from build123d import *

# Parameters (mm, degrees)
BOSS_EXTRUDE1_DEPTH = 5
SKETCH1_3_R         = 2.1
CUT_EXTRUDE1_DEPTH  = 57.124860802
SKETCH1_4_R         = 2.1
CUT_EXTRUDE2_DEPTH  = 57.124860802
SKETCH1_5_R         = 2.1
CUT_EXTRUDE3_DEPTH  = 57.124860802
SKETCH1_6_R         = 2.1
CUT_EXTRUDE4_DEPTH  = 57.124860802
BOSS_EXTRUDE2_DEPTH = 6
FILLET1_R           = 2
FILLET2_R           = 2
FILLET3_R           = 2
FILLET4_R           = 2
FILLET5_R           = 1


with BuildPart() as part:
    # Sketch1 → Boss-Extrude1 (new body)
    with BuildSketch(Plane(origin=(0, 0, 0), x_dir=(1, 0, 0), z_dir=(0, 1, 0))):
        with BuildLine():
            Line((-20, 0), (20, 0))
            ThreePointArc((20, 0), (23.535533906, -1.464466094), (25, -5))
            Line((25, -5), (25, -45))
            ThreePointArc((25, -45), (23.535533906, -48.535533906), (20, -50))
            Line((20, -50), (-20, -50))
            ThreePointArc((-20, -50), (-23.535533906, -48.535533906), (-25, -45))
            Line((-25, -45), (-25, -5))
            ThreePointArc((-25, -5), (-23.535533906, -1.464466094), (-20, 0))
        make_face()
    extrude(amount=BOSS_EXTRUDE1_DEPTH)

    # Sketch1_3 → Cut-Extrude1 (cut, through all)
    with BuildSketch(Plane(origin=(0, 0, 0), x_dir=(1, 0, 0), z_dir=(0, 1, 0))):
        with Locations(Location((20, -45, 0), (0, 0, 270))):
            Circle(SKETCH1_3_R)
    extrude(amount=CUT_EXTRUDE1_DEPTH, mode=Mode.SUBTRACT)

    # Sketch1_4 → Cut-Extrude2 (cut, through all)
    with BuildSketch(Plane(origin=(0, 0, 0), x_dir=(1, 0, 0), z_dir=(0, 1, 0))):
        with Locations(Location((20, -5, 0), (0, 0, 270))):
            Circle(SKETCH1_4_R)
    extrude(amount=CUT_EXTRUDE2_DEPTH, mode=Mode.SUBTRACT)

    # Sketch1_5 → Cut-Extrude3 (cut, through all)
    with BuildSketch(Plane(origin=(0, 0, 0), x_dir=(1, 0, 0), z_dir=(0, 1, 0))):
        with Locations(Location((-20, -5, 0), (0, 0, 90))):
            Circle(SKETCH1_5_R)
    extrude(amount=CUT_EXTRUDE3_DEPTH, mode=Mode.SUBTRACT)

    # Sketch1_6 → Cut-Extrude4 (cut, through all)
    with BuildSketch(Plane(origin=(0, 0, 0), x_dir=(1, 0, 0), z_dir=(0, 1, 0))):
        with Locations(Location((-20, -45, 0), (0, 0, 90))):
            Circle(SKETCH1_6_R)
    extrude(amount=CUT_EXTRUDE4_DEPTH, mode=Mode.SUBTRACT)

    # Sketch1_8 → Boss-Extrude2 (add)
    with BuildSketch(Plane(origin=(0, 0, 0), x_dir=(1, 0, 0), z_dir=(0, 1, 0))):
        with BuildLine():
            Line((17.051994501, -27.070918511), (17.051994501, -16.496039026))
            Line((17.051994501, -16.496039026), (20.029081489, -16.496039026))
            Line((20.029081489, -16.496039026), (20.029081489, -27.070918511))
            ThreePointArc((20.029081489, -27.070918511), (0, -47.1), (-20.029081489, -27.070918511))
            Line((-20.029081489, -27.070918511), (-20.029081489, -16.496039026))
            Line((-20.029081489, -16.496039026), (-17.051994501, -16.496039026))
            Line((-17.051994501, -16.496039026), (-17.051994501, -27.070918511))
            ThreePointArc((-17.051994501, -27.070918511), (0, -44.122913013), (17.051994501, -27.070918511))
        make_face()
    extrude(amount=-BOSS_EXTRUDE2_DEPTH)

    # Fillet1
    fillet1_edges = [part.edges().sort_by_distance(p)[0] for p in [
        (20.029081489, 0, 21.783478769),
        (-20.029081489, 0, 21.783478769),
        (0, 0, 47.1),
    ]]
    fillet(fillet1_edges, radius=FILLET1_R)

    # Fillet2
    fillet2_edges = [part.edges().sort_by_distance(p)[0] for p in [
        (17.051994501, -3, 16.496039026),
    ]]
    fillet(fillet2_edges, radius=FILLET2_R)

    # Fillet3
    fillet3_edges = [part.edges().sort_by_distance(p)[0] for p in [
        (-17.051994501, -3, 16.496039026),
    ]]
    fillet(fillet3_edges, radius=FILLET3_R)

    # Fillet4
    fillet4_edges = [part.edges().sort_by_distance(p)[0] for p in [
        (-20.029081489, -6, 21.783478769),
        (0, -6, 47.1),
        (20.029081489, -6, 21.783478769),
    ]]
    fillet(fillet4_edges, radius=FILLET4_R)

    # Fillet5
    fillet5_edges = [part.edges().sort_by_distance(p)[0] for p in [
        (0, 0, 0),
        (-23.535533906, 0, 1.464466094),
        (-25, 0, 25),
        (-23.535533906, 0, 48.535533906),
        (0, 0, 50),
        (23.535533906, 0, 48.535533906),
        (25, 0, 25),
        (23.535533906, 0, 1.464466094),
    ]]
    fillet(fillet5_edges, radius=FILLET5_R)


solid = part.part
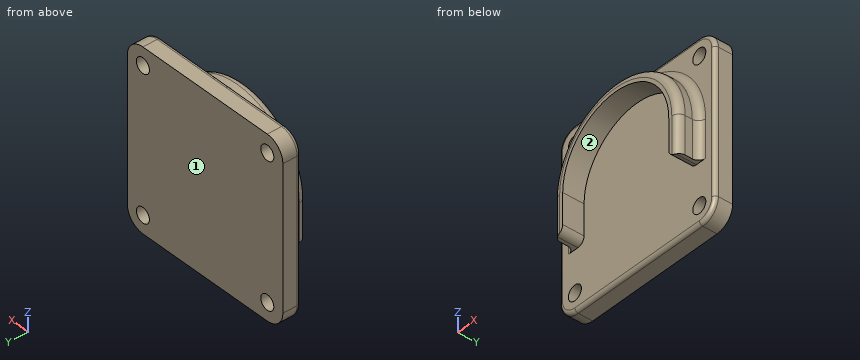
Read the model definition and answer for the solid it produces. Units are mm, in the model's axes. Face numbers are marked on the shaded views. Give positions to 0.01 mm unless a question says otherwise; leave off trailing zeros. Loops run counter-clockwise (first coordinate to the right, second up) from the corner with the lowest first, then second, coordinate; pieces in that order, holes last. Notation, with made-up numbers: (-14.5, 62) -> (14.5, 62) arc R31 cw to (14.5, 95) -> close; hole circle Ø10 at (0.25, 38). An arc over 180 degrees is marked (long way). Use a Markdown table: item, result.
Q1. Determine the mould class of the marked faces 1 and 2 for opening direction X: pulls with the +X half, pulls with the -X half, needs draft (parallel to the pull), parting line crosses it, or undercut.
Solved:
| item | result |
|---|---|
| face 1 | needs draft |
| face 2 | undercut |
Q2. Each of these flat-tipped pins is pushed along its axis until it touches: pin 1 (6.5 mm diameter, centred on y = -4.5, z = 22, fed in from +X); pin 2 (5.5 mm diameter, centred on x = 20, z = 5, fed in from +Y); pin 3 (2.5 mm diameter, centred on x = 20.5, y = -4, fed in from -Z); pin 4 (3 mm diameter, centred on x = 5, z = 23.5, fed in from -Y). Where does it stop, or does it pass through?
Solved:
| item | result |
|---|---|
| pin 1 | stops at x = 20.18 |
| pin 2 | stops at y = 5 |
| pin 3 | stops at z = 16.5 |
| pin 4 | stops at y = 0 |
Q3. Find the intervals of material crossed by line 1 along X through (y, z) = (3.9, 45); line 2 along Z through (x, y) = (-20, 1.5); line 3 along Y through (x, z) = (22, 48), in increasing order.
Solved:
| item | result |
|---|---|
| line 1 | x = -25 to -22.1, -17.9 to 17.9, 22.1 to 25 |
| line 2 | z = 0 to 2.9, 7.1 to 42.9, 47.1 to 50 |
| line 3 | y = 0 to 5 |
Q4. Section B-B, the plane z = 24 is taken. Determine the outline of the cut face in (x, y), then the cut area to 3 significant figures.
Solved:
| item | result |
|---|---|
| outline | (-25, 1) arc R1 ccw to (-24, 0) -> (-22.03, 0) arc R2 cw to (-20.03, -2) -> (-20.03, -4) arc R2 ccw to (-18.03, -6) -> (-17.05, -6) -> (-17.05, 0) -> (17.05, 0) -> (17.05, -6) -> (18.03, -6) arc R2 ccw to (20.03, -4) -> (20.03, -2) arc R2 cw to (22.03, 0) -> (24, 0) arc R1 ccw to (25, 1) -> (25, 5) -> (-25, 5) -> close |
| area | 285 mm^2 |
Q5. Section A-A, the plane y = 2.5 is taken. Determine the outline of the cut face in (x, z), then the cut area to 3 significant figures.
Solved:
| item | result |
|---|---|
| outline | (-25, 5) arc R5 ccw to (-20, 0) -> (20, 0) arc R5 ccw to (25, 5) -> (25, 45) arc R5 ccw to (20, 50) -> (-20, 50) arc R5 ccw to (-25, 45) -> close; hole circle Ø4.2 at (-20, 5); hole circle Ø4.2 at (-20, 45); hole circle Ø4.2 at (20, 5); hole circle Ø4.2 at (20, 45) |
| area | 2,420 mm^2 |
